from build123d import *

# Parameters (mm, degrees)
SKETCH1_W           = 25.4
SKETCH1_H           = 25.4
BOSS_EXTRUDE1_DEPTH = 241.3
SKETCH2_W           = 22.098
SKETCH2_H           = 22.098
CUT_EXTRUDE1_DEPTH  = 483.934094883


with BuildPart() as part:
    # Sketch1 → Boss-Extrude1 (new, symmetric)
    with BuildSketch(Plane(origin=(0, 0, 0), x_dir=(1, 0, 0), z_dir=(0, 1, 0))):
        Rectangle(SKETCH1_W, SKETCH1_H)
    extrude(amount=BOSS_EXTRUDE1_DEPTH, both=True)

    # Sketch2 → Cut-Extrude1 (cut, through all)
    with BuildSketch(Plane(origin=(0, 241.3, 0), x_dir=(1, 0, 0), z_dir=(0, 1, 0))):
        Rectangle(SKETCH2_W, SKETCH2_H)
    extrude(amount=-CUT_EXTRUDE1_DEPTH, mode=Mode.SUBTRACT)


solid = part.part
Check sheet for the modelled part. Datum: model origin and axes. Units: mm. A direction names the side the tool comes from. Round coordinates to 2 decimals unless told otherwise and drop trailing zeros. Loops run counter-clockwise (first coordinate to the right, second up) from the corner with the lowest first, then second, coordinate; pieces in that order, holes last. Notation, with made-up numbers: (-23.75, 73.25) -> (9.25, 73.25) arc R22 cw to (9.25, 92.25) -> close; hole circle Ø11 at (6, 24.25). An arc over 180 degrees is marked (long way). Put each result on its own line as item: value. Start each with the question number.
1. Section check B-B (z = 2.25). Enter the section's corners in (x, y), plus the area to 3 significant figures.
2. Scan line: probe 1 along Z at (x, y) = (6.5, -129.5). Record every from-to range of solid material in increasing order.
3. Section check A-A (x = -6.5). Enter the section's corners in (y, z).
4. Draft check along X on faces 3 (the face through (0, 3, -12.7)), 4 (the face through (12.7, 3, 0)), 5 (the face through (-11.049, 3, 0)). Enter one of: +X half, -X half, draft (parallel to the pull), parting line (faces both ways), or undercut.
5. Section check C-C (y = -161). Enter the section's corners in (x, z).
6. Access from +Z, -Z, +X, -X, +Y, -Y to the whole of each face (thin tool, end or side, straight path). Record for faces 1 (the face through (11.049, 3, 0)), 2 (the face through (-0.2, -241.3, -11.5)).
Findings:
1. outline: (-12.7, -241.3) -> (-11.05, -241.3) -> (-11.05, 241.3) -> (-12.7, 241.3) -> close; (11.05, -241.3) -> (12.7, -241.3) -> (12.7, 241.3) -> (11.05, 241.3) -> close
1. area: 1,590 mm^2
2. probe 1: z = -12.7 to -11.05, 11.05 to 12.7
3. outline: (-241.3, -12.7) -> (241.3, -12.7) -> (241.3, -11.05) -> (-241.3, -11.05) -> close; (-241.3, 11.05) -> (241.3, 11.05) -> (241.3, 12.7) -> (-241.3, 12.7) -> close
4. face 3: draft
4. face 4: +X half
4. face 5: undercut
5. outline: (-12.7, -12.7) -> (12.7, -12.7) -> (12.7, 12.7) -> (-12.7, 12.7) -> close; hole (-11.05, -11.05) -> (11.05, -11.05) -> (11.05, 11.05) -> (-11.05, 11.05) -> close
6. face 1: +Y, -Y
6. face 2: +Z, -Z, +X, -X, -Y
